```python
from build123d import *

# Parameters (mm, degrees)
F1_DEPTH = 300


with BuildPart() as f1:
    # F0 (on Front) → F1 (new body)
    with BuildSketch(Plane.XZ):
        Polygon((-51.054478, -4), (-75.054478, -4), (-75.054478, -5), (-50.377445, -5), (-42.377445, 15), (-22.439643, 15), (-14.439643, -5), (13.622555, -5), (21.622555, 15), (41.560357, 15), (49.560357, -5), (77.622555, -5), (85.622555, 15), (105.560357, 15), (113.560357, -5), (141.622555, -5), (149.622555, 15), (169.560357, 15), (176.303139, -1.856953), (177.231616, -1.485563), (170.23739, 16), (148.945522, 16), (140.945522, -4), (114.23739, -4), (106.23739, 16), (84.945522, 16), (76.945522, -4), (50.23739, -4), (42.23739, 16), (20.945522, 16), (12.945522, -4), (-13.76261, -4), (-21.76261, 16), (-43.054478, 16), align=None)
    extrude(amount=F1_DEPTH)


solid = f1.part
```
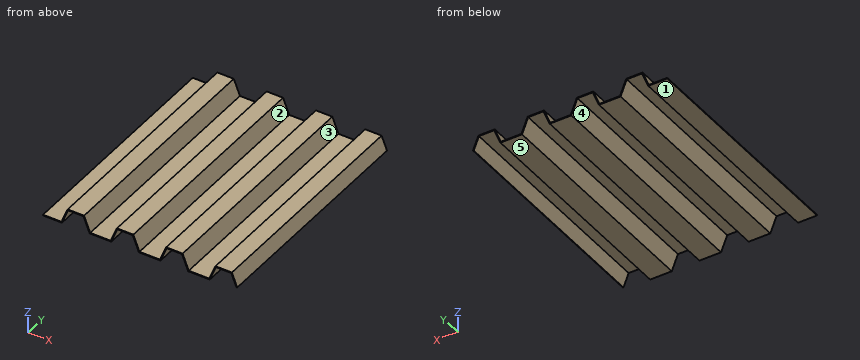
Can you work these out from the model? Positions are in its coordinate system, mm. Face numbers are marked on the shaded views. A direction names the side the tool comes from. Round coordinates to 2 decimals unless told otherwise and drop trailing zeros. Order: outer loops, then holes, each group sorted by start corner. A loop starts at its lowest first (then second) coordinate and runs counter-clockwise, first axis right, second up. Notation, with made-up numbers: (62, -33) -> (107, -33) arc R28 cw to (107, 5) -> close; hole circle Ø9 at (72.5, -12.75). An arc over 180 degrees is marked (long way). Return JSON: item names as keys, results as strings. Group by question number.
1. Will these pins go through, and if not, where does the flat tip stop? pin 1 (16 mm diameter, centred on x = 161.5, y = -156, fed in from -Z); pin 2 (21.5 mm diameter, centred on x = 68.5, y = -188, fed in from +Z); pin 3 (8 mm diameter, centred on x = 65, y = -112.5, fed in from +Z).
2. I need wall thicknesses on line 1 (Z direction, x = -2.5, y = -232); line 2 (Z direction, x = -28, y = -104.5). Which ranges of each line are inside material? Lowest first, please. Write a range as [from, to].
3. We'd pull the mould along X, two halves only. Please class the marked faces 1 and 2: released by +X, released by -X, zero draft, split by the parting line, or undercut.
4. If we section it at A-A, the plane z = 2: Count the separate pieces of the cut face and the enclosed holes in it, then the cut area to 3 significant figures.
5. If we section it at C-C, the plane x = 119: Write out the boundary of the cut face in (y, z).
6. Which directions (+Z, -Z, +X, -X, +Y, -Y) give clear straight access to the entire face, cutting with the end or side of a thin tool? Please do the marked faces 3, 4 and 5.
Output values:
{
 "1": {"pin 1": "z = 15", "pin 2": "z = 1.76", "pin 3": "z = -4"},
 "2": {"line 1": "[-5, -4]", "line 2": "[15, 16]"},
 "3": {"face 1": "zero draft", "face 2": "undercut"},
 "4": {"separate pieces": "8", "enclosed holes": "0", "area": "2,580 mm²"},
 "5": {"outline": "(-300, -5) -> (0, -5) -> (0, -4) -> (-300, -4) -> close"},
 "6": {"face 3": "+Z, +Y, -Y", "face 4": "-Z, +Y, -Y", "face 5": "-Z, +X, -X, +Y, -Y"}
}
